```python
from build123d import *

# Parameters (mm, degrees)
SKETCH2_R           = 1.5
SKETCH2_R_2         = 9.525
BOSS_EXTRUDE1_DEPTH = 4
BOSS_EXTRUDE2_START = 2.05
SKETCH2_4_R         = 9.525
SKETCH2_4_R_2       = 5.05
BOSS_EXTRUDE2_DEPTH = 1.95
SKETCH3_W           = 10
SKETCH3_H           = 30
BOSS_EXTRUDE3_DEPTH = 3
SKETCH4_R           = 2.525
CUT_EXTRUDE1_DEPTH  = 50.457052076
CHAMFER1_SIZE       = 10
FILLET2_R           = 1


with BuildPart() as part:
    # Sketch2 → Boss-Extrude1 (new, symmetric)
    with BuildSketch(Plane(origin=(0, 0, 0), x_dir=(0, 0, -1), z_dir=(1, 0, 0))):
        with BuildLine():
            Line((15, 0), (15, 30))
            ThreePointArc((15, 30), (0, 45), (-15, 30))
            Line((-15, 30), (-15, 0))
            Line((-15, 0), (15, 0))
        make_face()
        with Locations((-12, 30)):
            Circle(SKETCH2_R, mode=Mode.SUBTRACT)
        with Locations((0, 30)):
            Circle(SKETCH2_R_2, mode=Mode.SUBTRACT)
        with Locations((12, 30)):
            Circle(SKETCH2_R, mode=Mode.SUBTRACT)
    extrude(amount=BOSS_EXTRUDE1_DEPTH, both=True)

    # Sketch2<4> → Boss-Extrude2 (add)
    with BuildSketch(Plane(origin=(0, 0, 0), x_dir=(0, 0, -1), z_dir=(1, 0, 0)).offset(BOSS_EXTRUDE2_START)):
        with Locations((0, 30)):
            Circle(SKETCH2_4_R)
        with Locations((0, 30)):
            Circle(SKETCH2_4_R_2, mode=Mode.SUBTRACT)
    extrude(amount=BOSS_EXTRUDE2_DEPTH)

    # Sketch3 → Boss-Extrude3 (add)
    with BuildSketch(Plane.XZ):
        with Locations((9, 0)):
            Rectangle(SKETCH3_W, SKETCH3_H)
    extrude(amount=-BOSS_EXTRUDE3_DEPTH)

    # Sketch4 → Cut-Extrude1 (cut, through all)
    with BuildSketch(Plane(origin=(0, 0, 0), x_dir=(-1, 0, 0), z_dir=(0, -1, 0))):
        with Locations(Location((-8.964181233, 0, 0), (0, 0, 90))):
            Circle(SKETCH4_R)
    extrude(amount=-CUT_EXTRUDE1_DEPTH, mode=Mode.SUBTRACT)

    # Chamfer1
    chamfer1_edges = [part.edges().sort_by_distance(p)[0] for p in [
        (14, 1.5, -15),
        (14, 1.5, 15),
    ]]
    chamfer(chamfer1_edges, length=CHAMFER1_SIZE)

    # Fillet2
    fillet2_edges = [part.edges().sort_by_distance(p)[0] for p in [
        (4, 3, 0),
    ]]
    fillet(fillet2_edges, radius=FILLET2_R)


solid = part.part
```
Here's how the part is built. I have some questions about the finished solid (model axes, mm). A direction names the side the tool comes from. Coordinates: 2 decimals unless noted, no trailing zeros. Loops run counter-clockwise (first coordinate to the right, second up) from the corner with the lowest first, then second, coordinate; pieces in that order, holes last. Notation, with made-up numbers: (81.5, 49) - (139.5, 49) arc R17 cw to (139.5, 57) - close; hole circle Ø6 at (-31, 60.5). An arc over 180 degrees is marked (long way). Answer as CSV lines item,"result".
Q1. For pin 1 (15 mm diameter, centred on y = 34, z = 1.5, fed in from +X); pin 2 (6 mm diameter, centred on x = 8.96, z = 0, fed in from +Y); pin 3 (4 mm diameter, centred on x = 4, y = 36, fed in from -Z); pin 4 (6 mm diameter, centred on x = 4, z = -10, fed in from -Y), each with a flat end and sliding along its axis, tell me the tip position at first contact or that it passes through.
Response:
pin 1,"x = 4"
pin 2,"y = 3"
pin 3,"z = -14.46"
pin 4,"y = 0"
Q2. For faces 1 (the face through (-1.02, 20.7, 2.06)), 2 (the face through (6, 3, 0)), 3 (the face through (0, 15, -15)), which set-ups out of +Z, -Z, +X, -X, +Y, -Y let a thin tool reach every point of the face, with its end or its side?
Response:
face 1,"-X"
face 2,"+Z, -Z, +X, +Y"
face 3,"-Z, +X, -X, +Y, -Y"
Q3. If we section it at B-B, the plane z = 12: Write out the boundary of the cut face in (x, y).
Response:
outline,"(-4, 0) - (7, 0) - (7, 3) - (5, 3) arc R1 cw to (4, 4) - (4, 28.5) - (-4, 28.5) - close; (-4, 31.5) - (4, 31.5) - (4, 39) - (-4, 39) - close"
Q4. We'd pull the mould along Z, two halves only. Please class faces 4 (the face through (0, 45, 0)), 5 (the face through (2.05, 26, -4)), 6 (the face through (4, 24.8, 0.2)): pulls with the +Z half, pulls with the -Z half, needs draft (parallel to the pull), parting line crosses it, or undercut.
Response:
face 4,"parting line crosses it"
face 5,"undercut"
face 6,"needs draft"
Q5. If we section it at C-C, the plane x = 3.5: Write out the boundary of the cut face in (y, z), and give its area (3 significant figures).
Response:
outline,"(0, -15) - (30, -15) arc R15 ccw to (30, 15) - (0, 15) - close; hole circle Ø10.1 at (30, 0); hole circle Ø3 at (30, -12); hole circle Ø3 at (30, 12)"
area,"1,160 mm2"
Q6. If we section it at D-D, the plane y = 26: Write out the boundary of the cut face in (x, z), and give its area (3 significant figures).
Response:
outline,"(-4, -15) - (4, -15) - (4, -3.08) - (2.05, -3.08) - (2.05, -8.64) - (-4, -8.64) - close; (-4, 8.64) - (2.05, 8.64) - (2.05, 3.08) - (4, 3.08) - (4, 15) - (-4, 15) - close"
area,"123 mm2"
Q7. If we section it at A-A, the plane z = 0: Write out the boundary of the cut face in (x, y) (3 decimals).
Response:
outline,"(-4, 0) - (6.439, 0) - (6.439, 3) - (5, 3) arc R1 cw to (4, 4) - (4, 24.95) - (2.05, 24.95) - (2.05, 20.475) - (-4, 20.475) - close; (-4, 39.525) - (2.05, 39.525) - (2.05, 35.05) - (4, 35.05) - (4, 45) - (-4, 45) - close; (11.489, 0) - (14, 0) - (14, 3) - (11.489, 3) - close"
Q8. If I drill on L1, parallel to Y at x = 2.7, z = 0; L2, parallel to X at y = 4.5, z = 6; L3, parallel to X at y = 26.5, z = -7, over which ranges is the centre line in solid material (lowest first)? Write a range as [from, to].
Response:
L1,"[0, 24.95], [35.05, 45]"
L2,"[-4, 4]"
L3,"[2.05, 4]"
